Autodesk Inventor part; units mm, degrees
ref_plane "Work Plane1" through (0, 0, -70) normal (0, 0, 1) x (1, 0, 0)
ref_plane "YZ Plane" through (0, 0, 0) normal (1, 0, 0) x (0, 1, 0)
ref_plane "XZ Plane" through (0, 0, 0) normal (0, 1, 0) x (-1, 0, 0)
ref_plane "Work Plane1" through (0, 0, -70) normal (0, 0, 1) x (1, 0, 0)
sketch "Sketch1" plane through (0, 0, -70) normal (0, 0, 1) x (1, 0, 0)
  line L0 (105.135585, -0.094334) -> (105.135585, -23.278359)
  line L1 (-62.514415, -50.241251) -> (-62.514415, -27.759659)
  line L2 (-62.514415, -26.419466) -> (-62.514415, -51.782245)
  line L3 (102.485585, -0.094334) -> (102.485585, -23.278359)
  line L4 (102.485585, 1.408956) -> (105.135585, 1.408956)
  line L5 (-62.514415, -26.419466) -> (-62.514415, -51.782245)
  line L6 (-65.164415, -50.241251) -> (-65.164415, -27.759659)
  line L7 (-62.514415, -26.419466) -> (-65.164415, -26.419466)
  arc A0 (105.135585, 1.408956) -> (-65.164415, -26.419466) centre (24.560741, -40.503573) ccw
  line L8 (-65.164415, -26.419466) -> (-67.161965, -26.419466)
  arc A1 (102.485585, 1.408956) -> (-62.514415, -26.419466) centre (24.895442, -41.61673) ccw
  line L9 (-65.164415, -26.419466) -> (-69.658457, -26.419466)
  arc A2 (-34.319919, 30.819568) -> (-69.658457, -26.419466) centre (14.828678, -39.052317) ccw
  line L10 (-34.319919, 30.819568) -> (-32.803901, 29.911365)
  line L11 (105.135585, 1.408956) -> (107.351745, 3.413316)
  arc A3 (107.351745, 3.413316) -> (70.831931, 40.201852) centre (31.896127, -34.970341) ccw
  line L12 (70.831931, 40.201852) -> (69.891547, 38.198928)
  line L13 (102.485585, 1.408956) -> (102.485585, -2.185128)
  line L14 (102.485585, -2.185128) -> (105.135585, -2.185128)
  line L15 (107.351745, 3.413316) -> (105.135585, -2.185128)
  line L16 (-69.658457, -26.419466) -> (-65.164415, -34.970341)
  line L17 (-65.164415, -34.970341) -> (-62.514415, -34.970341)
  line L18 (-62.514415, -34.970341) -> (-62.514415, -26.419466)
  point P0 (0, 0)
  point P1 (-31.670702, 30.819568)
extrude "Extrusion1" add sketch "Sketch1" along normal blind 25.4
fillet "Fillet1" radius 12.7 4 edges at (-33.5619, 30.3655, -70) (-33.5619, 30.3655, -44.6) (70.3617, 39.2004, -70) (70.3617, 39.2004, -44.6)
properties part number "thigh_strap_01" material "Acetal Resin, Black"
The model under review builds one solid part; all positions refer to its coordinate system, in mm. A direction names the side the tool comes from. Coordinates: 2 decimals unless noted, no trailing zeros. Order: outer loops, then holes, each group sorted by start corner. A loop starts at its lowest first (then second) coordinate and runs counter-clockwise, first axis right, second up. Notation, with made-up numbers: (-0.75, 7.25) -> (31.25, 7.25) arc R22 cw to (31.25, 46.25) -> close; hole circle Ø3 at (41, 84.5). An arc over 180 degrees is marked (long way). Answer in a Markdown table with one row per item. Add a question column.
Item 1: We need section A-A on y = 7. Write out the cut boundary in (x, z).
Item 2: We need section D-D on y = -18. Write out the cut boundary in (x, z).
Item 3: We need section B-B on z = -53.75. Write out the cut boundary in (x, y), plus the area to 3 significant figures.
Item 4: Machinability: for faces 1 (the cylindrical face through (73.405, 37.161, -66.181)), 2 (the flat face through (-62.514, -31, -57)), 3 (the flat face through (102.486, 0, -57)), 4 (the cylindrical face through (-37.05, 27.53, -47.84)), which of the approach directions +Z, -Z, +X, -X, +Y, -Y give a long, thin tool a straight path to every point of the face, cutting with its end or side? Answer none if there is none.
Item 5: We need section C-C on x = -49.5. Write out the cut boundary in (y, z), plus the area to 3 significant figures.
Item 6: To check wall thickness, follow probe 1 along X at (y, z) = (37, -47.5); probe 2 along X at (y, z) = (26, -53); probe 3 along X at (y, z) = (22.5, -56.75). State the ranges of each line that lie inside material, in increasing order.
Item 7: Mouldability with a two-part tool opening along X and no side actions: class faces 5 (the cylindrical face through (8.63, 45.6, -57.48)), 6 (the flat face through (5, 46, -44.6)), 7 (the cylindrical face through (91.72, 24.93, -57.48)) as +X half, -X half, draft (parallel to the pull), parting line (faces both ways), or undercut.
Item 8: Clearance check with flat-ended pins moving along their axes: pin 1 (1.3 mm diameter, centred on x = 103.5, z = -53.5, fed in from -Y); pin 2 (1 mm diameter, centred on x = 78.5, y = 34, fed in from +Z); pin 3 (4.5 mm diameter, centred on y = -31.5, z = -62.5, fed in from +X). State where each tip first meets the part, or that it passes through.
Final values:
| question | item | result |
|---|---|---|
| 1 | outline | (-57.12, -70) -> (-49.32, -70) -> (-49.32, -44.6) -> (-57.12, -44.6) -> close; (99.11, -70) -> (105.42, -70) -> (105.42, -44.6) -> (99.11, -44.6) -> close |
| 2 | outline | (-67.96, -70) -> (-60.62, -70) -> (-60.62, -44.6) -> (-67.96, -44.6) -> close |
| 3 | outline | (-69.66, -26.42) -> (-65.16, -34.97) -> (-62.51, -34.97) -> (-62.51, -26.42) arc R88.72 cw to (102.49, 1.41) -> (102.49, -2.19) -> (105.14, -2.19) -> (107.35, 3.41) arc R84.66 ccw to (71.28, 39.97) -> (70.33, 37.94) arc R90.82 ccw to (-33.22, 29.57) -> (-34.77, 30.5) arc R85.43 ccw to start |
| 3 | area | 1,100 mm2 |
| 4 | face 1 | -Z, +Y |
| 4 | face 2 | +Z, -Z, +X, -Y |
| 4 | face 3 | +Z, -Z, -Y |
| 4 | face 4 | +Z, +Y |
| 5 | outline | (6.72, -70) -> (17.16, -70) -> (17.16, -44.6) -> (6.72, -44.6) -> close |
| 5 | area | 265 mm2 |
| 6 | probe 1 | x = -22.79 to -16.22, 66.02 to 71.91, 74.43 to 76.47 |
| 6 | probe 2 | x = -40.54 to -32.55, 82.34 to 90.63 |
| 6 | probe 3 | x = -44.41 to -36.43, 86.22 to 94.06 |
| 7 | face 5 | undercut |
| 7 | face 6 | draft |
| 7 | face 7 | +X half |
| 8 | pin 1 | stops at y = -2.19 |
| 8 | pin 2 | stops at z = -44.87 |
| 8 | pin 3 | stops at x = -62.51 |
